Source: three-view drawing plus pictorial views. Frame: mm from the lowest corner of the part. A direction names the side the tool comes from. Round coordinates to 2 decimals unless told otherwise and drop trailing zeros. Loops run counter-clockwise (first coordinate to the right, second up) from the corner with the lowest first, then second, coordinate; pieces in that order, holes last. Notation, with made-up numbers: (-24.75, 48.5) -> (-16.75, 48.5) arc R26 cw to (-16.75, 83.5) -> close; hole circle Ø6 at (72, -5). An arc over 180 degrees is marked (long way). Answer in a Markdown table with one row per item. Add a question column.
Q1. Reachability of the marked faces 1, 2 and 3 from +Z, -Z, +X, -X, +Y, -Y: full face, straight path, thin tool, end or side. Return the list, or none.
Q2. Section D-D, the plane y = 59. Output: boundary loops of the cut face in (x, z).
Q3. Ray query, L1, parallel to X at y = 74, z = 12.5; L2, parallel to Y at x = 49.5, z = 5; L3, parallel to Y at x = 14, z = 4.5. Return the intervals inside material, ascending. Write a range as from..to.
Q4. Section C-C, the plane z = 4.75. Output: boundary loops of the cut face in (x, y), and give its area (3 significant figures).
Q5. Section B-B, the plane x = 39. Output: boundary loops of the cut face in (y, z).
Q6. Section A-A, the plane y = 76.5. Output: boundary loops of the cut face in (x, z), and give its area (3 significant figures).
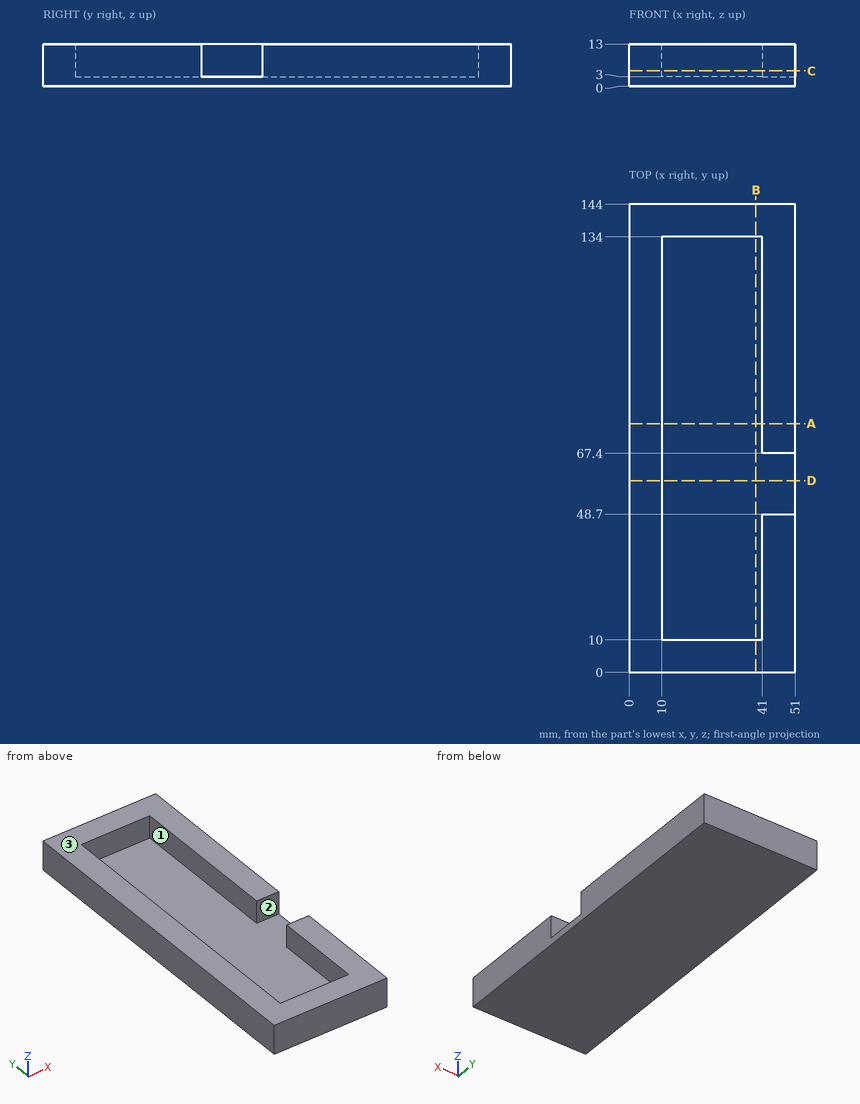
Answer block:
| question | item | result |
|---|---|---|
| 1 | face 1 | +Z |
| 1 | face 2 | +Z, +X |
| 1 | face 3 | +Z, +X, -X, +Y, -Y |
| 2 | outline | (0, 0) -> (51, 0) -> (51, 3) -> (10, 3) -> (10, 13) -> (0, 13) -> close |
| 3 | L1 | 0..10, 41..51 |
| 3 | L2 | 0..48.7, 67.4..144 |
| 3 | L3 | 0..10, 134..144 |
| 4 | outline | (0, 0) -> (51, 0) -> (51, 48.7) -> (41, 48.7) -> (41, 10) -> (10, 10) -> (10, 134) -> (41, 134) -> (41, 67.4) -> (51, 67.4) -> (51, 144) -> (0, 144) -> close |
| 4 | area | 3,310 mm^2 |
| 5 | outline | (0, 0) -> (144, 0) -> (144, 13) -> (134, 13) -> (134, 3) -> (10, 3) -> (10, 13) -> (0, 13) -> close |
| 6 | outline | (0, 0) -> (51, 0) -> (51, 13) -> (41, 13) -> (41, 3) -> (10, 3) -> (10, 13) -> (0, 13) -> close |
| 6 | area | 353 mm^2 |
